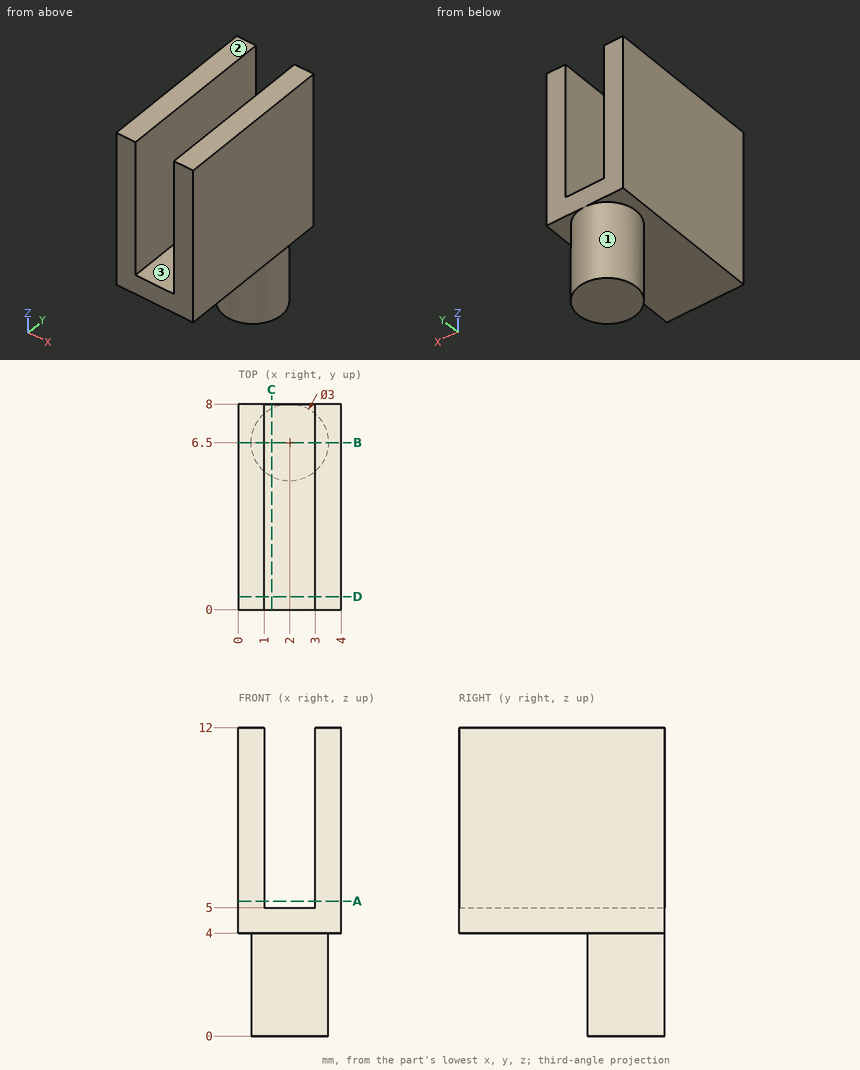
Source: three-view drawing plus pictorial views. Frame: mm from the lowest corner of the part. A direction names the side the tool comes from. Give positions to 0.01 mm unless a question says otherwise; leave off trailing zeros. Order: outer loops, then holes, each group sorted by start corner. A loop starts at its lowest first (then second) coordinate and runs counter-clockwise, first axis right, second up. Notation, with made-up numbers: M 35,10.5 L 65,10.5 A20 ccw 65,31.5 Z; hole C 83,-20.5 d5. An arc over 180 degrees is marked long. Return JSON: item names as keys, results as strings.
Item 1: Ray query, probe 1 along X at (y, z) = (7.75, 9); probe 2 along Z at (x, y) = (1.6, 5.75); probe 3 along Z at (x, y) = (0.25, 7.25). Return the intervals inside material, ascending.
Solutions:
{"probe 1": "0 to 1, 3 to 4", "probe 2": "0 to 5", "probe 3": "4 to 12"}
Item 2: Cut plane C-C (x = 1.3). Return loops of the section in (y, z).
Solutions:
{"outline": "M 0,4 L 5.17,4 L 5.17,0 L 7.83,0 L 7.83,4 L 8,4 L 8,5 L 0,5 Z"}
Item 3: Access query for the marked faces 1, 2 and 3. Directions: +Z, -Z, +X, -X, +Y, -Y. A direction counts if a zero-diameter tool reaches every point of the face in a straight line with its end or side. Return the directions, or none.
Solutions:
{"face 1": "-Z", "face 2": "+Z, +X, -X, +Y, -Y", "face 3": "+Z, +Y, -Y"}
Item 4: First-contact query: P1, Ø2, axis at x = 1.5, z = 9, coming from the -Y side. Flat tip, straight axial feed; report the tip coordinate or a pass-through.
Solutions:
{"P1": "y = 0"}
Item 5: Cut plane D-D (y = 0.5). Return loops of the section in (x, z).
Solutions:
{"outline": "M 0,4 L 4,4 L 4,12 L 3,12 L 3,5 L 1,5 L 1,12 L 0,12 Z"}
Item 6: Cut plane B-B (y = 6.5). Return loops of the section in (x, z).
Solutions:
{"outline": "M 0,4 L 0.5,4 L 0.5,0 L 3.5,0 L 3.5,4 L 4,4 L 4,12 L 3,12 L 3,5 L 1,5 L 1,12 L 0,12 Z"}
Item 7: Cut plane A-A (z = 5.25). Return loops of the section in (x, y).
Solutions:
{"outline": "M 0,0 L 1,0 L 1,8 L 0,8 Z; M 3,0 L 4,0 L 4,8 L 3,8 Z"}
